Geometry check sheet. Reference: drawing and pictorial views, mm from the part's lowest x, y, z. Round coordinates to 2 decimals unless told otherwise and drop trailing zeros. Order: outer loops, then holes, each group sorted by start corner. A loop starts at its lowest first (then second) coordinate and runs counter-clockwise, first axis right, second up.
(1) Gauge pin test, flat end, axial feed: P1, Ø6, axis at x = 24.5, y = 45, coming from the -Z side. Record the tip position at first contact, or that the pin passes through.
(2) Thickness scan on L1, parallel to X at y = 1.75, z = 6.35; L2, parallel to X at y = 52, z = 8.5; L3, parallel to Z at x = 19.05, y = 66.25. Record the ranges inside material, lowest first.
(3) Cross-section at A-A on y = 12.5. Enter the section's corners in (x, z).
(4) Cross-section at C-C on z = 6.35. Count the separate pieces of the cut face and the enclosed holes in it, and give its area (3 significant figures).
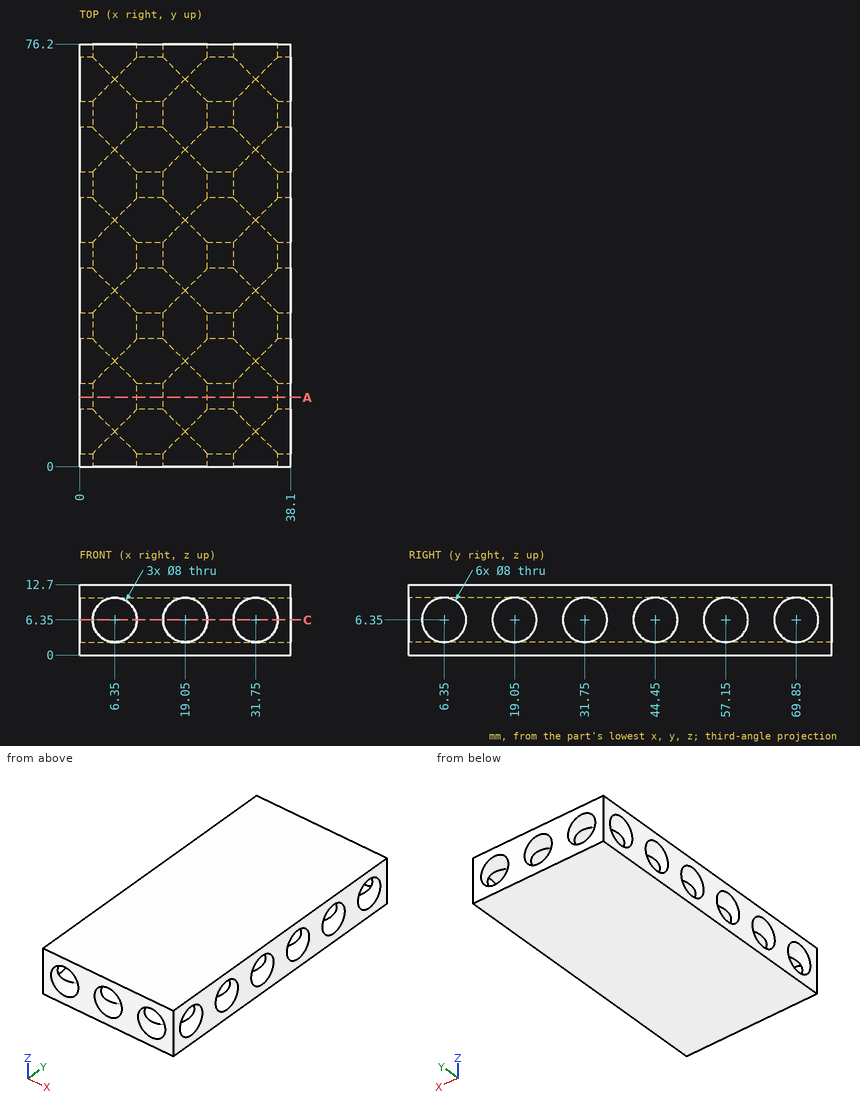
Found:
1. P1: stops at z = 0
2. L1: x = 0 to 2.35, 10.35 to 15.05, 23.05 to 27.75, 35.75 to 38.1
2. L2: x = 0 to 2.98, 9.72 to 15.68, 22.42 to 28.38, 35.12 to 38.1
2. L3: z = 0 to 2.35, 10.35 to 12.7
3. outline: (0, 0) - (38.1, 0) - (38.1, 12.7) - (0, 12.7) - close; hole circle Ø8 at (6.35, 6.35); hole circle Ø8 at (19.05, 6.35); hole circle Ø8 at (31.75, 6.35)
4. separate pieces: 28
4. enclosed holes: 0
4. area: 398 mm2
